Can you work these out from the model? Positions are in its coordinate system, mm. A direction names the side the tool comes from. Give positions to 0.01 mm unless a question says otherwise; leave off trailing zeros. Loops run counter-clockwise (first coordinate to the right, second up) from the corner with the lowest first, then second, coordinate; pieces in that order, holes last. Notation, with made-up numbers: (-31, 8.5) -> (26, 8.5) arc R20 ccw to (26, 12.5) -> close; hole circle Ø5 at (57.25, 19). An arc over 180 degrees is marked (long way). Use CSV: the item, a comma, the result in double quotes.
from build123d import *

# Parameters (mm, degrees)
SKETCH16_W                                     = 25.4
SKETCH16_H                                     = 25.4
SKETCH16_W_2                                   = 22.098
SKETCH16_H_2                                   = 22.098
AL_TUBE_SQUARE_AL_TUBE_1_SQR_X_0_065_WAL_DEPTH = 615.4
F_1_4_0_25_DIAMETER_HOLE1_D                    = 6.35


with BuildPart() as part:
    # Sketch16 → Al tube square AL TUBE 1 SQR X 0.065 WALL(1) (new body)
    with BuildSketch(Plane(origin=(0, 0, 0), x_dir=(0, 0, -1), z_dir=(1, 0, 0))):
        Rectangle(SKETCH16_W, SKETCH16_H)
        Rectangle(SKETCH16_W_2, SKETCH16_H_2, mode=Mode.SUBTRACT)
    extrude(amount=AL_TUBE_SQUARE_AL_TUBE_1_SQR_X_0_065_WAL_DEPTH)

    # 1/4 (0.25) Diameter Hole1 (through all)
    with Locations(Plane(origin=(0, 12.7, 0), x_dir=(1, 0, 0), z_dir=(0, 1, 0))):
        with Locations((466.45, 0), (148.95, 0)):
            Hole(F_1_4_0_25_DIAMETER_HOLE1_D / 2)


solid = part.part
(1) If I drill on L1, parallel to Z at x = 148.95, y = -12.2 (3 decimals); L2, parallel to Y at x = 434, z = -8.5, over which ranges is the centre line in solid material (lowest first)? Write a range as from..to.
Answer sheet:
L1,"z = -12.7..-3.175, 3.175..12.7"
L2,"y = -12.7..-11.05, 11.05..12.7"
(2) We'd pull the mould along Z, two halves only. Please class faces 1 (the face through (303, 0, 12.7)), 2 (the face through (303, 0, -12.7)), 3 (the face through (303, -11.049, 0)): released by +Z, released by -Z, zero draft, split by the parting line, or undercut.
Answer sheet:
face 1,"released by +Z"
face 2,"released by -Z"
face 3,"undercut"
(3) Which directions (+Z, -Z, +X, -X, +Y, -Y) give clear straight access to the entire face, cutting with the end or side of a thin tool? Please do faces 4 (the face through (303, 11.049, 0)), 5 (the face through (303, 12.7, 0)).
Answer sheet:
face 4,"+X, -X"
face 5,"+Z, -Z, +X, -X, +Y"
(4) Will this pin go through, and if not, where does the flat tip stop? pin 1 Ø5 at (x, z) = (466.45, 0) entering from +Y.
Answer sheet:
pin 1,"passes through"
(5) If we section it at B-B, the plane y = 2: Write out the boundary of the cut face in (x, z).
Answer sheet:
outline,"(0, -12.7) -> (615.4, -12.7) -> (615.4, -11.05) -> (0, -11.05) -> close; (0, 11.05) -> (615.4, 11.05) -> (615.4, 12.7) -> (0, 12.7) -> close"
(6) If we section it at A-A, the plane x = 544: Write out the boundary of the cut face in (y, z), then the cut area to 3 significant figures.
Answer sheet:
outline,"(-12.7, -12.7) -> (12.7, -12.7) -> (12.7, 12.7) -> (-12.7, 12.7) -> close; hole (-11.05, -11.05) -> (11.05, -11.05) -> (11.05, 11.05) -> (-11.05, 11.05) -> close"
area,"157 mm2"
